Work out the finished part from the listing and answer in its coordinate system (mm). Face numbers are marked on the shaded views. A direction names the side the tool comes from. Coordinates: 2 decimals unless noted, no trailing zeros. Loops run counter-clockwise (first coordinate to the right, second up) from the corner with the lowest first, then second, coordinate; pieces in that order, holes last. Notation, with made-up numbers: (73, -4) -> (131, -4) arc R13 ccw to (131, 11) -> close; hole circle Ø11 at (-11, -31). An arc over 180 degrees is marked (long way). One line per question, with ' | ' between items.
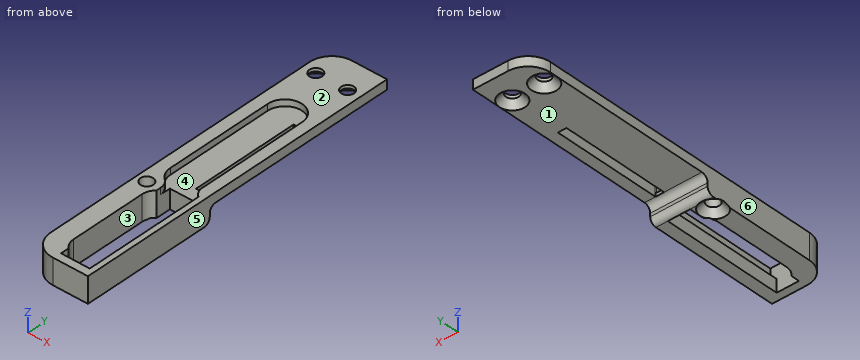
Autodesk Inventor part; units mm, degrees
ref_plane "YZ Plane" through (0, 0, 0) normal (1, 0, 0) x (0, 1, 0)
ref_plane "XZ Plane" through (0, 0, 0) normal (0, 1, 0) x (-1, 0, 0)
ref_plane "XY Plane" through (0, 0, 0) normal (0, 0, 1) x (1, 0, 0)
sketch "草图1" plane through (0, 0, 0) normal (0, 0, 1) x (1, 0, 0)
  point P0 (0, 0)
sketch "草图2" plane through (0, 0, 0) normal (0, 0, 1) x (1, 0, 0)
  arc A0 (-0.8636, -19.593) -> (1.5364, -19.593) centre (0.3364, -19.593) ccw
  line L0 (-0.8636, -19.593) -> (-0.8636, -7.593)
  arc A1 (1.5364, -7.593) -> (-0.8636, -7.593) centre (0.3364, -7.593) ccw
  line L1 (1.5364, -7.593) -> (1.5364, -19.593)
  arc A2 (-1.8636, -1.5566) -> (1.5364, -1.5566) centre (-0.1636, -1.5566) ccw
  line L2 (-1.8636, 15.4434) -> (-1.8636, -1.5566)
  arc A3 (1.5364, 15.4434) -> (-1.8636, 15.4434) centre (-0.1636, 15.4434) ccw
  line L3 (1.5364, 8.4451) -> (1.5364, 15.4434)
  arc A4 (1.3364, 8.2451) -> (1.5364, 8.4451) centre (1.3364, 8.4451) ccw
  line L4 (1.3364, 8.2451) -> (1.2785, 8.2451)
  arc A5 (1.0785, 8.4451) -> (1.2785, 8.2451) centre (1.2785, 8.4451) ccw
  line L5 (1.0785, 8.4451) -> (1.0785, 15.3461)
  arc A6 (1.0785, 15.3461) -> (-1.3205, 15.3461) centre (-0.121, 15.3461) ccw
  line L6 (-1.3205, 15.3461) -> (-1.3205, -1.4976)
  arc A7 (-1.3205, -1.4976) -> (1.0785, -1.4976) centre (-0.121, -1.4976) ccw
  line L7 (1.0785, -1.4976) -> (1.0785, 5.4033)
  arc A8 (1.2785, 5.6033) -> (1.0785, 5.4033) centre (1.2785, 5.4033) ccw
  line L8 (1.2785, 5.6033) -> (1.3364, 5.6033)
  arc A9 (1.5364, 5.4033) -> (1.3364, 5.6033) centre (1.3364, 5.4033) ccw
  line L9 (1.5364, -1.5566) -> (1.5364, 5.4033)
  arc A10 (-4.7477, -20.3592) -> (-3.3007, -23.1939) centre (-1.2477, -20.3592) ccw
  spline S0 degree 3 poles (-1.2477, -23.8592) (-1.6067, -23.8592) (-1.9735, -23.8009) (-2.735, -23.5583) (-3.0595, -23.3686) (-3.3007, -23.1939) knots 0 0 0 0 0.450925 0.450925 1 1 1 1
  line L10 (5.2523, -23.8592) -> (-1.2477, -23.8592)
  line L11 (5.2523, 28.3531) -> (5.2523, -23.8592)
  line L12 (-1.2477, 28.3531) -> (5.2523, 28.3531)
  arc A11 (-1.2477, 28.3531) -> (-4.7477, 24.8531) centre (-1.2477, 24.8531) ccw
  line L13 (-4.7477, -20.3592) -> (-4.7477, 24.8531)
  line L14 (4.2523, -23.8592) -> (4.2523, 28.3531)
  line L15 (5.2523, 28.3531) -> (4.2523, 28.3531)
  line L16 (5.2523, -23.8592) -> (5.2523, 28.3531)
  line L17 (4.2523, -23.8592) -> (5.2523, -23.8592)
  point P0 (0, 0)
extrude "拉伸1" add sketch "草图2" along normal blind 4 contours L0 A1 L1 A0 | L2 A3 L3 A4 L4 A5 L5 A6 L6 A7 L7 A8 L8 A9 L9 A2 | L13 A11 L12 L14 L10 S0 A10
sketch "草图3" plane through (0, 0, 4) normal (0, 0, 1) x (1, 0, 0)
  point P0 (0, 0)
sketch "草图4" plane through (0, 0, 0) normal (0, 0, -1) x (-1, 0, 0)
  line L0 (-3.3928, -22.593) -> (-3.3928, -3.4829)
  line L1 (-3.3928, -3.4829) -> (-4.2523, -3.4829)
  line L2 (-4.2523, -3.4829) -> (-4.2523, -23.8592)
  line L3 (-4.2523, -23.8592) -> (1.2477, -23.8592)
  spline S0 degree 3 poles (1.2477, -23.8592) (1.6878, -23.8592) (2.1571, -23.7712) (2.6422, -23.5699) (2.6953, -23.5463) (2.7477, -23.5215) knots 0 0 0 0 0.889543 0.889543 1 1 1 1
  line L4 (2.7477, -23.5215) -> (2.7477, -3.4829)
  line L5 (2.7477, -3.4829) -> (1.1072, -3.4829)
  line L6 (1.1072, -3.4829) -> (1.1072, -5.9329)
  arc A0 (1.8636, -7.593) -> (1.1072, -5.9329) centre (-0.3364, -7.593) ccw
  line L7 (1.8636, -7.593) -> (1.8636, -19.593)
  arc A1 (1.1072, -21.2531) -> (1.8636, -19.593) centre (-0.3364, -19.593) ccw
  line L8 (1.1072, -21.2531) -> (1.1072, -22.593)
  line L9 (1.1072, -22.593) -> (-3.3928, -22.593)
  line L10 (1.1072, -3.593) -> (-3.3928, -3.593)
  point P0 (0, 0)
extrude "拉伸2" cut sketch "草图4" against normal blind 4 contours L0 L10 L6 A0 L7 A1 L8 L9
sketch "草图5" plane through (0, 0, 0) normal (0, 0, -1) x (-1, 0, 0)
  line L0 (-2.3928, -3.593) -> (-2.3928, -22.593)
  line L1 (-2.3928, -3.593) -> (-3.3928, -3.593)
  line L2 (-3.3928, -22.593) -> (-3.3928, -3.593)
  line L3 (-2.3928, -22.593) -> (-3.3928, -22.593)
  point P0 (0, 0)
extrude "拉伸3" add sketch "草图5" against normal blind 2
sketch "草图6" plane through (4.2523, -23.8592, 0) normal (1, 0, 0) x (0, 0, -1)
  line L0 (0.0883, 54.0026) -> (-2.5, 54.0026)
  line L1 (-2.5, 54.0026) -> (-2.5, 21.2662)
  line L2 (-2.5, 21.2662) -> (0.0883, 21.2662)
  line L3 (0.0883, 21.2662) -> (0.0883, 54.0026)
  line L4 (1, 20.2662) -> (-3, 20.2662)
  line L5 (-4, 0) -> (-4, 52.2123)
  point P0 (0, 23.8592)
  point P1 (-1, 20.2662)
  dimension "d6" = 1
  dimension "d7" = 1.5
extrude "拉伸4" cut sketch "草图6" against normal blind 33
fillet "圆角1" radius 1 2 edges at (-0.2477, -2.593, 2.5) (-0.2477, -2.593, 0)
sketch "草图7" plane through (0, 0, 4) normal (0, 0, 1) x (1, 0, 0)
  arc A0 (-1.8636, -1.5566) -> (1.5364, -1.5566) centre (-0.1636, -1.5566) ccw
  line L0 (-1.8636, 15.4434) -> (-1.8636, -1.5566)
  line L1 (1.5364, -1.5566) -> (1.5364, 5.4033)
  line L2 (1.379, -1.5758) -> (1.379, 15.4242)
  arc A1 (1.5364, 15.4434) -> (-1.8636, 15.4434) centre (-0.1636, 15.4434) ccw
  line L3 (1.5364, -1.5566) -> (1.5364, 15.4434)
  line L4 (-2.8636, 15.4434) -> (-2.8636, -1.5566)
  arc A2 (-2.8636, -1.5566) -> (2.5364, -1.5566) centre (-0.1636, -1.5566) ccw
  line L5 (2.5364, -1.5566) -> (2.5364, 15.4434)
  arc A3 (2.5364, 15.4434) -> (-2.8636, 15.4434) centre (-0.1636, 15.4434) ccw
  point P0 (0, 0)
  dimension "d11" = 1
extrude "拉伸5" cut sketch "草图7" against normal blind 1 contours L0 A1 L3 L1 A0 | A3 L5 A2 L4
fillet "圆角2" radius 2 2 edges at (-1.1072, -4.0864, 3.5) (1.6093, -3.593, 3.5)
sketch "草图8" plane through (0, 0, 3) normal (0, 0, 1) x (1, 0, 0)
  arc A0 (2.5364, 15.4434) -> (-2.8636, 15.4434) centre (-0.1636, 15.4434) ccw
  line L0 (2.5364, 15.4434) -> (1.1862, 15.4434)
  line L1 (1.1862, 15.4434) -> (1.1862, -1.593)
  line L2 (1.1862, -1.593) -> (2.5364, -1.593)
  line L3 (2.5364, -1.593) -> (2.5364, 15.4434)
  line L4 (-4.7477, -1.593) -> (4.2523, -1.593)
  point P0 (0, 0)
extrude "拉伸6" cut sketch "草图8" against normal blind 1
sketch "草图9" plane through (0, 0, 4) normal (0, 0, 1) x (1, 0, 0)
  point P0 (0, 0)
sketch "草图10" plane through (0, 0, 4) normal (0, 0, 1) x (1, 0, 0)
  circle A0 centre (-2.7477, 23.7142) radius 1
  circle A1 centre (2.2523, 23.7142) radius 1
  line L0 (4.2523, -23.8592) -> (4.2523, 28.3531)
  line L1 (-4.7477, 24.8531) -> (-4.7477, -20.3592)
  circle A2 centre (-3.1277, -5.3622) radius 1
  point P0 (0, 0)
  dimension "d17" = 2
  dimension "d18" = 2
  dimension "d19" = 2
  dimension "d20" = 2
  dimension "d21" = 2
extrude "拉伸7" cut sketch "草图10" against normal blind 9.5
chamfer "倒角1" distance 1 angle 45 3 edges at (-3.7477, 23.7142, 2.5) (1.2523, 23.7142, 2.5) (-4.1277, -5.3622, 0)
properties part number "指纹安装板"
1) Flat-ended cylindrical pins translate along their axes: pin 1 (1.5 mm diameter, centred on y = 5, z = 1.5, fed in from -X); pin 2 (1.5 mm diameter, centred on x = -2.5, z = 2.5, fed in from +Y); pin 3 (4.5 mm diameter, centred on x = 1, y = 15, fed in from -Z); pin 4 (2 mm diameter, centred on x = -0.5, z = 0.5, fed in from +Y). Find the tip coordinate at first contact, or state that the pin passes through.
Check values:
pin 1: passes through | pin 2: stops at y = 28.32 | pin 3: stops at z = 2.5 | pin 4: stops at y = -2.59
2) The mould has two halves that part along X. Classify the marked faces 3, 4, 5 and 6: released by +X, released by -X, zero draft, split by the parting line, or undercut.
Check values:
face 3: undercut | face 4: undercut | face 5: released by +X | face 6: released by -X
3) Find the intervals of material crossed by line 1 along X through (y, z) = (-10, 2.3); line 2 along Y through (x, z) = (0.5, 1.2); line 3 along X through (y, z) = (11, 2.95), in increasing order.
Check values:
line 1: x = -4.75 to -1.86, 3.39 to 4.25 | line 2: y = -23.86 to -22.59, -3.59 to -2.59 | line 3: x = -4.75 to 1.19, 2.54 to 4.25
4) Find section A-A (y = 5). Write down the section's boundary in (x, z).
Check values:
outline: (-4.75, 2.5) -> (1.19, 2.5) -> (1.19, 3) -> (-2.86, 3) -> (-2.86, 4) -> (-4.75, 4) -> close; (2.54, 2.5) -> (4.25, 2.5) -> (4.25, 4) -> (2.54, 4) -> close
5) For the marked faces 1 and 2, determine the directions among +Z, -Z, +X, -X, +Y, -Y from which every point of the face is accessible in a straight line to the end or side of a thin tool.
Check values:
face 1: -Z, +X, -X, +Y | face 2: +Z, +X, -X, +Y, -Y
